Solid Edge part; units mm, degrees
sketch "Sketch1" plane through (0, 0, 0) normal (0, -1, 0) x (1, 0, 0)
  line L0 (4, 0) -> (15, 0)
  line L1 (15, 0) -> (15, 6)
  line L2 (15, 6) -> (5.5, 6)
  line L3 (5.5, 6.5) -> (5.5, 6)
  line L4 (4, 6.5) -> (5.5, 6.5)
  line L5 (4, 6.5) -> (4, 0)
revolve "RevolvedProtrusion1" add sketch "Sketch1" angle 360 about axis through (0, 0, 6.5) along (0, 0, -1)
sketch "Sketch2" plane through (0, 0, 6) normal (0, 0, 1) x (1, 0, 0)
  line L0 (14.4568, -4) -> (5.5, 0)
  line L1 (5.5, 0) -> (4.0445, 9.0396)
  line L2 (-5.5, 0) -> (-3.84, 9.12)
  line L3 (-14.4568, -4) -> (-5.5, 0)
  line L4 (-14.4568, -4) -> (-19.3107, 1.4462)
  line L5 (-19.3107, 1.4462) -> (-10.4784, 15.4995)
  line L6 (-10.4784, 15.4995) -> (15.0272, 16.6485)
  line L7 (15.0272, 16.6485) -> (21.6119, 7.3238)
  line L8 (21.6119, 7.3238) -> (21.1258, -3.415)
  line L9 (21.1258, -3.415) -> (14.4568, -4)
  arc A0 (4.0445, 9.0396) -> (-3.84, 9.12) centre (0.0953, 8.4037) ccw
  circle A1 centre (0, 8) radius 2
extrude "Cutout1" cut sketch "Sketch2" along normal through all and the other way through all
hole "Bohrung_1" at (0, 0, 3) direction (0, -1, 0) diameter 3.242 end up to next thread major 4 thread length 2
Work out the finished part from the listing and answer in its coordinate system (mm). A direction names the side the tool comes from. Round coordinates to 2 decimals unless told otherwise and drop trailing zeros. Write each loop counter-clockwise with the first axis right and the second up, starting at its lowest first coordinate (ties: lowest second). Pieces come first, ordered by that corner, then holes. Notation, with made-up numbers: (78, 13) - (87, 13) arc R20 ccw to (87, 38) - close; hole circle Ø6 at (36.25, 39). An arc over 180 degrees is marked (long way). Answer in a Markdown table with one row per item. Add a question column.
1. Find the intervals of material crossed by line 1 along Z through (x, y) = (0, -11); line 2 along Y through (x, z) = (0, 2.3); line 3 along Z through (x, y) = (-12.75, -6.75), in increasing order. Write a range as from..to.
2. A cutting plane is placed at B-B, the plane y = -1.5. Determine the outline of the cut face in (x, z), and give its area (3 significant figures).
3. A cutting plane is placed at D-D, the plane y = -7.5. Determine the outline of the cut face in (x, z).
4. For faces 4 (the cylindrical face through (0.1, -5.5, 6.2)), 5 (the flat face through (4.78, 4.46, 3.2)), 6 (the cylindrical face through (0, 5.5, 6.2)), determine the directions among +Z, -Z, +X, -X, +Y, -Y from which every point of the face is accessible in a straight line to the end or side of a thin tool.
5. A cutting plane is placed at C-C, the plane x = 0. Determine the outline of the cut face in (y, z), and give its area (3 significant figures).
6. Given pin 1 (3 mm diameter, centred on y = 5.5, z = 4, fed in from -X); pin 2 (2 mm diameter, centred on y = 8, z = 3.5, fed in from +X); pin 3 (6 mm diameter, centred on x = 10, y = -9.5, fed in from +Z), each flat-ended and moving along its own axis, determine where each tip first touches the part or whether it passes through.
7. A cutting plane is placed at A-A, the plane z = 1. Count the separate pieces of the cut face and the enclosed holes in it, and give its area (3 significant figures).
8. The mould has two halves that part along Z. Classify faces 1 (the cylindrical face through (0.058, 12.404, 2.958)), 2 (the cylindrical face through (-0.986, -9.249, 1.714)), 3 (the flat face through (2, 4, 6.5)): +Z half, -Z half, draft (parallel to the pull), parting line (faces both ways), or undercut.
Worked out:
| question | item | result |
|---|---|---|
| 1 | line 1 | 0..1.38, 4.62..6 |
| 1 | line 2 | 4..6, 10..12.4 |
| 1 | line 3 | 0..6 |
| 2 | outline | (-8.86, 0) - (-3.71, 0) - (-3.71, 6.5) - (-5.29, 6.5) - (-5.29, 6) - (-8.86, 6) - close; (3.71, 0) - (8.86, 0) - (8.86, 6) - (5.29, 6) - (5.29, 6.5) - (3.71, 6.5) - close |
| 2 | area | 63.4 mm^2 |
| 3 | outline | (-12.99, 0) - (12.99, 0) - (12.99, 6) - (-12.99, 6) - close; hole circle Ø3.24 at (0, 3) |
| 4 | face 4 | +Z, -Y |
| 4 | face 5 | +Z, -Z, +X, +Y |
| 4 | face 6 | +Z, +Y |
| 5 | outline | (-15, 0) - (-4, 0) - (-4, 1.38) - (-15, 1.38) - close; (-15, 4.62) - (-4, 4.62) - (-4, 6.5) - (-5.5, 6.5) - (-5.5, 6) - (-15, 6) - close; (4, 0) - (6, 0) - (6, 6) - (5.5, 6) - (5.5, 6.5) - (4, 6.5) - close; (10, 0) - (12.4, 0) - (12.4, 6) - (10, 6) - close |
| 5 | area | 58.3 mm^2 |
| 6 | pin 1 | x = -4.77 |
| 6 | pin 2 | x = 4.37 |
| 6 | pin 3 | z = 6 |
| 7 | separate pieces | 1 |
| 7 | enclosed holes | 2 |
| 7 | area | 357 mm^2 |
| 8 | face 1 | draft |
| 8 | face 2 | undercut |
| 8 | face 3 | +Z half |
